Can you work these out from the model? Positions are in its coordinate system, mm. Face numbers are marked on the shaded views. A direction names the side the tool comes from. Round coordinates to 2 decimals unless told otherwise and drop trailing zeros. Loops run counter-clockwise (first coordinate to the right, second up) from the corner with the lowest first, then second, coordinate; pieces in that order, holes last. Notation, with made-up numbers: M -10,-5 L 31,-5 A23 ccw 31,16 Z; hole C 15.25,4 d11. An arc over 180 degrees is marked long. Return JSON: item names as keys, results as strings.
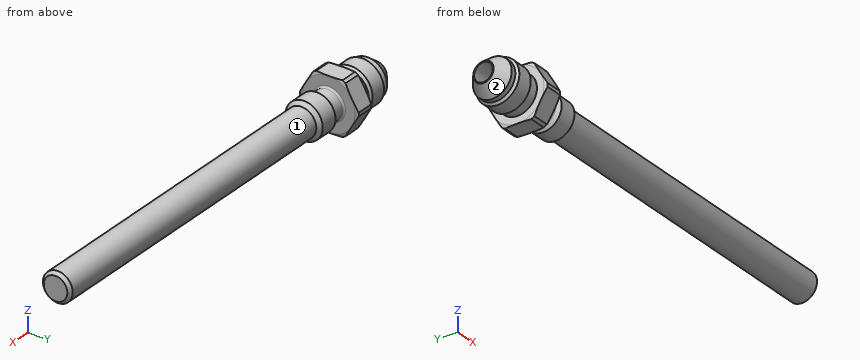
```python
from build123d import *

# Parameters (mm, degrees)
SKETCH_2_OUTSIDE_W  = 49.708
SKETCH_2_OUTSIDE_H  = 49.708
CUT_EXTRUDE_1_DEPTH = 127
CHAMFER_1_SIZE      = 1
FILLET_1_R          = 0.6


with BuildPart() as part:
    # Эскиз1 → Повернуть1 (revolve)
    with BuildSketch(Plane.XY):
        Polygon((0, 8.5), (0, 4.8), (4, 4.8), (5.2, 6), (10.8, 6), (12, 4.8), (120, 4.8), (120, 0), (115.802581857, 0), (114, 3), (-21, 3), (-21, 3.3), (-17.085217776, 6.25), (-15.5, 6.25), (-14.75, 7), (-9.75, 7), (-9, 6.25), (-6, 6.25), (-6, 8.5), (-5.732050808, 9.5), (-0.267949192, 9.5), align=None)
    revolve(axis=Axis((0, 0, 0), (-1, 0, 0)))

    # Эскиз2 outside → Вырез-Вытянуть1 (cut, through all)
    with BuildSketch(Plane.ZY.offset(6)):
        Rectangle(SKETCH_2_OUTSIDE_W, SKETCH_2_OUTSIDE_H)
        Polygon((0, 9.814954576), (-8.5, 4.907477288), (-8.5, -4.907477288), (0, -9.814954576), (8.5, -4.907477288), (8.5, 4.907477288), align=None, mode=Mode.SUBTRACT)
    extrude(amount=-CUT_EXTRUDE_1_DEPTH, mode=Mode.SUBTRACT)

    # Фаска1
    chamfer_1_edges = [part.edges().sort_by_distance(p)[0] for p in [
        (120, -4.8, 0),
    ]]
    chamfer(chamfer_1_edges, length=CHAMFER_1_SIZE)

    # Скругление1
    fillet_1_edges = [part.edges().sort_by_distance(p)[0] for p in [
        (4, -4.8, 0),
        (0, -4.8, 0),
    ]]
    fillet(fillet_1_edges, radius=FILLET_1_R)


solid = part.part
```
Q1. On a 3-axis mill with a long thin cutter (end or side, diameter ignored), from which of +Z, -Z, +X, -X, +Y, -Y can I reach the whole of each face in a straight line? I mean the marked faces 1 and 2. Say none if no direction works.
Results:
{"face 1": "+X", "face 2": "-X"}
Q2. If I drill on line 1 along Z through (x, y) = (75, 0); line 2 along Y through (x, z) = (6, 2.5), over which ranges is the centre line in solid material (lowest first)?
Results:
{"line 1": "z = -4.8 to -3, 3 to 4.8", "line 2": "y = -5.45 to -1.66, 1.66 to 5.45"}
Q3. Suppose I cut it at A-A, the plane x = 78. Please give me the cut outline in (y, z).
Results:
{"outline": "C 0,0 d9.6; hole C 0,0 d6"}
Q4. I'm going to push flat-ended pins straight in: pin 1 Ø1.5 at (x, y) = (10.5, 0.5) entering from +Z; pin 2 Ø2 at (y, z) = (-2, 4) entering from -X; pin 3 Ø6 at (x, z) = (101, 0) entering from -Y. Where does each tip first touch, or does it pass through?
Results:
{"pin 1": "stops at z = 6", "pin 2": "stops at x = -20.77", "pin 3": "stops at y = -4.8"}
